Part model, mm, in its own coordinate system. A direction names the side the tool comes from. Round coordinates to 2 decimals unless told otherwise and drop trailing zeros. Write each loop counter-clockwise with the first axis right and the second up, starting at its lowest first coordinate (ties: lowest second). Pieces come first, ordered by that corner, then holes.
1) Saw through at D-D on z = -35. Write the cut outline in (x, y).
2) Which spindle directions (+Z, -Z, +X, -X, +Y, -Y) get a long thin tool onto all of the face, cutting with end or side? Do faces 4 (the cylindrical face through (21.49, 1.97, -28.01)), 5 (the flat face through (36, 2, 22)), 6 (the flat face through (-26, 2, 0)). Say none if no direction does.
3) Pull direction X, two halves, no side cores. Call faces 1 (the cylindrical face through (-10.195, 1.972, -15.587)), 2 (the flat face through (26, 2, 0)), 3 (the cylindrical face through (0.781, 1.972, -49.994)): +X half, -X half, draft (parallel to the pull), parting line (faces both ways), or undercut.
4) Saw through at C-C on x = -22.6. Write the cut outline in (y, z).
5) Saw through at B-B on y = 2.4. Count the separate pieces of the cut face and the enclosed holes in it, and give its area (3 significant figures).
6) Flat gauge pins, fed straight in: pin 1 (2 mm diameter, centred on x = 32.5, y = 2.5, fed in from +Z); pin 2 (1.9 mm diameter, centred on x = 0, z = 27.7, fed in from -Y); pin 3 (1 mm diameter, centred on x = 31, y = 1, fed in from +Z); pin 4 (1 mm diameter, centred on y = 1, z = -33.5, fed in from -X). Where does each tip first touch, or does it go through?
7) Drill centre lines: L1, parallel to X at y = 3.2, z = 14.1; L2, parallel to Z at x = 0, y = 2.8; L3, parallel to X at y = 2.1, z = 27. Where is each one in solid material? Low to high.
8) Saw through at A-A on z = 14.1. Write the cut outline in (x, y), and give its area (3 significant figures).
```python
from build123d import *

# Parameters (mm, degrees)
SKETCH1_R           = 1.5
SKETCH1_R_2         = 1.6
SKETCH1_R_3         = 7.5
BOSS_EXTRUDE1_DEPTH = 4


with BuildPart() as part:
    # Sketch1 → Boss-Extrude1 (new body)
    with BuildSketch(Plane(origin=(0, 0, 0), x_dir=(1, 0, 0), z_dir=(0, 1, 0))):
        with BuildLine():
            Line((-44.899888641, 22), (-26, 22))
            Line((-26, 22), (-26, -22))
            Line((-26, -22), (-44.899888641, -22))
            ThreePointArc((-44.899888641, -22), (0, -50), (44.899888641, -22))
            Line((44.899888641, -22), (26, -22))
            Line((26, -22), (26, 22))
            Line((26, 22), (44.899888641, 22))
            ThreePointArc((44.899888641, 22), (0, 50), (-44.899888641, 22))
        make_face()
        with Locations((-22.6, -41)):
            Circle(SKETCH1_R, mode=Mode.SUBTRACT)
        with Locations((-22.6, -27)):
            Circle(SKETCH1_R, mode=Mode.SUBTRACT)
        with Locations((-10, -14.1)):
            Circle(SKETCH1_R, mode=Mode.SUBTRACT)
        with Locations((0, -27.7)):
            Circle(SKETCH1_R_2, mode=Mode.SUBTRACT)
        with Locations((22.6, -41)):
            Circle(SKETCH1_R, mode=Mode.SUBTRACT)
        with Locations((22.6, -27)):
            Circle(SKETCH1_R, mode=Mode.SUBTRACT)
        with Locations((10, -14.1)):
            Circle(SKETCH1_R, mode=Mode.SUBTRACT)
        with Locations((-10, 14.1)):
            Circle(SKETCH1_R, mode=Mode.SUBTRACT)
        with Locations((-22.6, 27)):
            Circle(SKETCH1_R, mode=Mode.SUBTRACT)
        with Locations((-22.6, 41)):
            Circle(SKETCH1_R, mode=Mode.SUBTRACT)
        with Locations((0, 40)):
            Circle(SKETCH1_R_3, mode=Mode.SUBTRACT)
        with Locations((10, 14.1)):
            Circle(SKETCH1_R, mode=Mode.SUBTRACT)
        with Locations((0, 27.7)):
            Circle(SKETCH1_R_2, mode=Mode.SUBTRACT)
        with Locations((22.6, 27)):
            Circle(SKETCH1_R, mode=Mode.SUBTRACT)
        with Locations((22.6, 41)):
            Circle(SKETCH1_R, mode=Mode.SUBTRACT)
    extrude(amount=BOSS_EXTRUDE1_DEPTH)


solid = part.part
```
Completed:
1. outline: (-35.71, 0) - (-5.59, 0) - (-5.59, 4) - (-35.71, 4) - close; (5.59, 0) - (35.71, 0) - (35.71, 4) - (5.59, 4) - close
2. face 4: +Y, -Y
2. face 5: +X, +Y, -Y
2. face 6: -X, +Y, -Y
3. face 1: undercut
3. face 2: +X half
3. face 3: parting line
4. outline: (0, -44.6) - (4, -44.6) - (4, -42.5) - (0, -42.5) - close; (0, -39.5) - (4, -39.5) - (4, -28.5) - (0, -28.5) - close; (0, -25.5) - (4, -25.5) - (4, 25.5) - (0, 25.5) - close; (0, 28.5) - (4, 28.5) - (4, 39.5) - (0, 39.5) - close; (0, 42.5) - (4, 42.5) - (4, 44.6) - (0, 44.6) - close
5. separate pieces: 1
5. enclosed holes: 15
5. area: 5,610 mm2
6. pin 1: stops at z = 38.83
6. pin 2: passes through
6. pin 3: stops at z = 39.62
6. pin 4: stops at x = -37.56
7. L1: x = -26 to -11.5, -8.5 to 8.5, 11.5 to 26
7. L2: z = -50 to -47.5, -32.5 to -29.3, -26.1 to 26.1, 29.3 to 50
7. L3: x = -42.08 to -24.1, -21.1 to -1.44, 1.44 to 21.1, 24.1 to 42.08
8. outline: (-26, 0) - (-11.5, 0) - (-11.5, 4) - (-26, 4) - close; (-8.5, 0) - (8.5, 0) - (8.5, 4) - (-8.5, 4) - close; (11.5, 0) - (26, 0) - (26, 4) - (11.5, 4) - close
8. area: 184 mm2
